Print and shaded views of the part. All mm, measured from the part's lowest x, y and z. A direction names the side the tool comes from. Round coordinates to 2 decimals unless told otherwise and drop trailing zeros. Write each loop counter-clockwise with the first axis right and the second up, starting at its lowest first coordinate (ties: lowest second). Pieces come first, ordered by that corner, then holes. Notation, with made-up numbers: (-3.5, -23) - (27.5, -23) arc R35 ccw to (27.5, 11) - close; hole circle Ø7 at (50.5, 47). An arc over 180 degrees is marked (long way). Put each result on its own line as item: value. Start each with the question number.
Item 1: 3-axis set-ups, long thin cutter, end or side, ignore diameter. For the marked faces 1 and 2: which of +Z, -Z, +X, -X, +Y, -Y reach the whole face in a straight line?
Item 2: Pin check, flat tips, straight feed: pin 1 Ø4 at (x, z) = (30.53, 19.135) entering from -Y; pin 2 Ø12 at (x, z) = (5, 4.5) entering from -Y; pin 3 Ø0.8 at (x, y) = (18, 1) entering from +Z; pin 4 Ø1.5 at (x, z) = (19.5, 11.5) entering from +Y. Stop position of each tip, or through.
Item 3: Mould opens along X. For the marked faces 3, 4, 5 and 6 say: released by +X, released by -X, zero draft, split by the parting line, or undercut.
Item 4: Cut at B-B (x = 25.5). Give the cut face in (y, z).
Item 5: Cut at A-A (z = 14). Give the cut face in (x, y), and give its area (3 significant figures).
Item 6: Drill centre lines: line 1 (X direction, y = 2, z = 4.5); line 2 (Z direction, x = 29.5, y = 2.8) (1 decimal); line 3 (X direction, y = 1.6, z = 9) (1 decimal). Where is each one in solid material? Low to high. Write a range as from..to.
Item 7: Cut at D-D (y = 0.85). Give the cut face in (x, z), and give its area (3 significant figures).
Item 8: Cut at C-C (y = 2.4). Give the cut face in (x, z) (1 decimal).
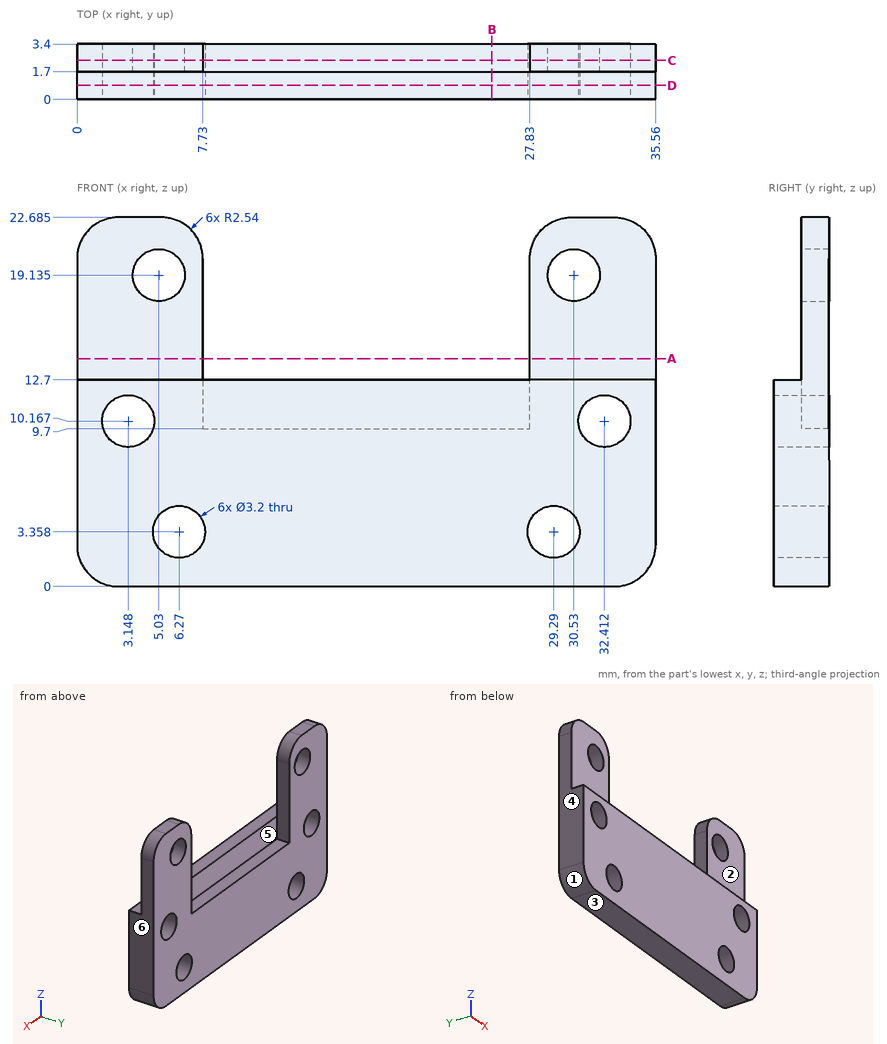
Output values:
1. face 1: -Z, -X, +Y, -Y
1. face 2: +Z, +X, -X, -Y
2. pin 1: y = 1.7
2. pin 2: y = 0
2. pin 3: z = 12.7
2. pin 4: y = 1.7
3. face 3: zero draft
3. face 4: released by -X
3. face 5: undercut
3. face 6: released by +X
4. outline: (0, 0) - (3.4, 0) - (3.4, 9.7) - (1.7, 9.7) - (1.7, 12.7) - (0, 12.7) - close
5. outline: (0, 1.7) - (7.73, 1.7) - (7.73, 3.4) - (0, 3.4) - close; (27.83, 1.7) - (35.56, 1.7) - (35.56, 3.4) - (27.83, 3.4) - close
5. area: 26.3 mm2
6. line 1: 0..5.15, 7.39..28.17, 30.41..35.56
6. line 2: 0..1.8, 4.9..17.9, 20.4..22.5
6. line 3: 0..2.1, 4.2..31.3, 33.5..35.6
7. outline: (0, 2.54) arc R2.54 ccw to (2.54, 0) - (33.02, 0) arc R2.54 ccw to (35.56, 2.54) - (35.56, 12.7) - (0, 12.7) - close; hole circle Ø3.2 at (3.15, 10.17); hole circle Ø3.2 at (6.27, 3.36); hole circle Ø3.2 at (29.29, 3.36); hole circle Ø3.2 at (32.41, 10.17)
7. area: 417 mm2
8. outline: (0, 2.5) arc R2.5 ccw to (2.5, 0) - (33, 0) arc R2.5 ccw to (35.6, 2.5) - (35.6, 20.1) arc R2.5 ccw to (33, 22.7) - (30.4, 22.7) arc R2.5 ccw to (27.8, 20.1) - (27.8, 9.7) - (7.7, 9.7) - (7.7, 20.1) arc R2.5 ccw to (5.2, 22.7) - (2.5, 22.7) arc R2.5 ccw to (0, 20.1) - close; hole circle Ø3.2 at (3.1, 10.2); hole circle Ø3.2 at (5, 19.1); hole circle Ø3.2 at (6.3, 3.4); hole circle Ø3.2 at (29.3, 3.4); hole circle Ø3.2 at (30.5, 19.1); hole circle Ø3.2 at (32.4, 10.2)
